```python
from build123d import *

# Parameters (mm, degrees)
F15_DEPTH = 16.5
F16_R     = 20.5
F17_DEPTH = 16.5
F18_R     = 4.0274870607
F19_DEPTH = 16.5
F20_W     = 3
F20_H     = 20
F21_DEPTH = 16.5
F22_R     = 2.75
F23_DEPTH = 40
F26_DEPTH = 31.3
F27_R     = 22.25
F28_DEPTH = 5
F29_R     = 1
F30_R     = 5
F31_R     = 5
F32_R     = 5
F33_R     = 5
F34_R     = 5
F35_R     = 2
F36_R     = 2


# Not quite as in the source:
# - a feature of the source that left no trace in its solid (it failed there, or was rolled back) is left out


with BuildPart() as f15:
    # F14 (on offset) → F15 (new body)
    with BuildSketch(Plane.XZ.offset(20)):
        Polygon((8.5, 39.5), (-8.5, 39.5365608335), (-56.3052967191, -10.4271536693), (-56.1165139079, -24.8827897012), (-50.9412027895, -33.6846895516), (12.0133129929, -33.5), (12.0133129929, -27.1025877446), (22.7434113622, -16.4029654115), (27.6456046849, 0), (22.3432332277, 17.5122059882), (8.5, 25.806048885), align=None)
    extrude(amount=F15_DEPTH)

    # F16 (on face) → F17 (cut)
    with BuildSketch(Plane.XZ.offset(36.5)):
        Circle(F16_R)
    extrude(amount=-F17_DEPTH, mode=Mode.SUBTRACT)

    # F18 (on face) → F19 (cut)
    with BuildSketch(Plane.XZ.offset(36.5)):
        with Locations((-45.0200997293, -24.5124399662)):
            Circle(F18_R)
    extrude(amount=-F19_DEPTH, mode=Mode.SUBTRACT)

    # F20 (on face) → F21 (cut)
    with BuildSketch(Plane.XZ.offset(36.5)):
        with Locations((0, 30.4450483003)):
            Rectangle(F20_W, F20_H)
    extrude(amount=-F21_DEPTH, mode=Mode.SUBTRACT)

    # F22 (on face) → F23 (cut)
    with BuildSketch(Plane.YZ.offset(8.5)):
        with Locations((-29, 32.35)):
            Circle(F22_R)
    extrude(amount=-F23_DEPTH, mode=Mode.SUBTRACT)

    # F25 (on offset) → F26 (cut)
    with BuildSketch(Plane.YZ.offset(-36.7)):
        Polygon((-32.875, 34.5872322931), (-32.875, 30.1127677069), (-29, 27.8755354138), (-25.125, 30.1127677069), (-25.125, 34.5872322931), (-29, 36.8244645862), align=None)
    extrude(amount=F26_DEPTH, mode=Mode.SUBTRACT)

    # F27 (on face) → F28 (cut)
    with BuildSketch(Plane.XZ.offset(36.5)):
        Circle(F27_R)
    extrude(amount=-F28_DEPTH, mode=Mode.SUBTRACT)

    # F29
    f29_edges = [f15.edges().sort_by_distance(p)[0] for p in [
        (-49.047587, -36.5, -24.51244),
        (-1.5, -20, 29.983277),
        (1.5, -20, 29.980051),
        (-1.5, -34, 22.199381),
        (-1.5, -31.5, 21.322214),
        (-1.5, -25.75, 20.445048),
        (1.5, -25.75, 20.445048),
        (1.5, -31.5, 21.322214),
        (1.5, -34, 22.199381),
    ]]
    fillet(f29_edges, radius=F29_R)

    # F30
    f30_edges = [f15.edges().sort_by_distance(p)[0] for p in [
        (27.645605, -28.25, 0),
    ]]
    fillet(f30_edges, radius=F30_R)

    # F31
    f31_edges = [f15.edges().sort_by_distance(p)[0] for p in [
        (22.343233, -28.25, 17.512206),
    ]]
    fillet(f31_edges, radius=F31_R)

    # F32
    f32_edges = [f15.edges().sort_by_distance(p)[0] for p in [
        (22.743411, -28.25, -16.402965),
    ]]
    fillet(f32_edges, radius=F32_R)

    # F33
    f33_edges = [f15.edges().sort_by_distance(p)[0] for p in [
        (8.5, -28.25, 25.806049),
    ]]
    fillet(f33_edges, radius=F33_R)

    # F34
    f34_edges = [f15.edges().sort_by_distance(p)[0] for p in [
        (-50.941203, -28.25, -33.68469),
        (-56.116514, -28.25, -24.88279),
        (-56.305297, -28.25, -10.427154),
    ]]
    fillet(f34_edges, radius=F34_R)

    # F35
    f35_edges = [f15.edges().sort_by_distance(p)[0] for p in [
        (12.013313, -28.25, -33.5),
        (12.013313, -28.25, -27.102588),
    ]]
    fillet(f35_edges, radius=F35_R)

    # F36
    f36_edges = [f15.edges().sort_by_distance(p)[0] for p in [
        (-8.5, -28.25, 39.536561),
        (8.5, -28.25, 39.5),
    ]]
    fillet(f36_edges, radius=F36_R)


solid = f15.part
```
Source: CAD feature listing. Evaluate the final solid. Frame: model axes, mm. A direction names the side the tool comes from. Round coordinates to 2 decimals unless told otherwise and drop trailing zeros. Write each loop counter-clockwise with the first axis right and the second up, starting at its lowest first coordinate (ties: lowest second). Pieces come first, ordered by that corner, then holes. Notation, with made-up numbers: M -3.75,62 L 43.25,62 A28 cw 43.25,95 Z; hole C 57,-14 d4. An arc over 180 degrees is marked long. Answer as a JSON object with one key per item and string values. Group by question number.
(1) Ray query, line 1 (X direction, y = -32.75, z = 34.5); line 2 (Y direction, x = 6, z = 32); line 3 (Z direction, x = -3.65, y = -29). Return the intervals inside material, ascending. Write a range as [from, to].
(2) First-contact query: pin 1 (1 mm diameter, centred on x = 10.5, y = -27.5, fed in from -Z); pin 2 (3 mm diameter, centred on y = -23, z = 0.5, fed in from +X); pin 3 (2 mm diameter, centred on y = -29.5, z = -1, fed in from -X); pin 4 (9 mm diameter, centred on y = -29, z = 32.35, fed in from +X). Flat tips, straight axial feed; report the tip coordinate or a pass-through.
(3) Reachability of faces 5 (the flat face through (-8.5, -30.91, 35.72)), 6 (the flat face through (15.877, -28.134, 21.386)), 7 (the cylindrical face through (-0.94, -34.03, -22.23)) from +Z, -Z, +X, -X, +Y, -Y: full face, straight path, thin tool, end or side. Return the list, or none.
(4) Section query A-A on x = -6.5. Output: boundary loops of the cut face in (y, z) (3 decimals).
(5) Mould query, pull axis Y, two halves, no side actions, for faces 1 (the flat face through (-8.502, -27.035, 35.69)), 2 (the cylindrical face through (27.424, -28.366, 0.02)), 3 (the flat face through (-24, -36.5, -5)), 4 (the cylindrical face through (5.049, -31.747, 32.471)). Classes: +Y half, -Y half, draft (parallel to the pull), parting line (faces both ways), or undercut.
(6) Section query B-B on z = 0. Output: boundary loops of the cut face in (x, y).
(7) Section query C-C on z = 32.35. Output: boundary loops of the cut face in (x, y) (3 decimals), then the cut area to 3 significant figures.
Computed values:
{
 "1": {"line 1": "[-5.4, -1.5], [1.5, 8.5]", "line 2": "[-36.5, -31.73], [-26.27, -20]", "line 3": "[-33.55, -20.17], [20.17, 29.6], [35.1, 39.53]"},
 "2": {"pin 1": "z = -33.51", "pin 2": "x = 27.42", "pin 3": "x = -48.24", "pin 4": "x = 8.56"},
 "3": {"face 5": "-X", "face 6": "+Z, +X, +Y, -Y", "face 7": "-Y"},
 "4": {"outline": "M -36.5,-33.554 L -20,-33.554 L -20,-19.442 L -31.5,-19.442 L -31.5,-21.279 L -36.5,-21.279 Z; M -36.5,21.279 L -31.5,21.279 L -31.5,19.442 L -20,19.442 L -20,39.532 L -36.5,39.532 Z; hole M -32.875,30.113 L -29,27.876 L -25.125,30.113 L -25.125,34.587 L -29,36.824 L -32.875,34.587 Z"},
 "5": {"face 1": "undercut", "face 2": "draft", "face 3": "-Y half", "face 4": "undercut"},
 "6": {"outline": "M -46.33,-36.5 L -22.25,-36.5 L -22.25,-31.5 L -20.5,-31.5 L -20.5,-20 L -46.33,-20 Z; M 20.5,-31.5 L 22.25,-31.5 L 22.25,-36.5 L 27.42,-36.5 L 27.42,-20 L 20.5,-20 Z"},
 "7": {"outline": "M -15.376,-36.5 L -1.5,-36.5 L -1.5,-31.75 L -5.4,-31.75 L -5.4,-32.875 L -15.376,-32.875 Z; M -15.376,-25.125 L -5.4,-25.125 L -5.4,-26.25 L -1.5,-26.25 L -1.5,-21 A1 ccw -2.5,-20 L -15.376,-20 Z; M 1.5,-36.5 L 8.5,-36.5 L 8.5,-31.75 L 1.5,-31.75 Z; M 1.5,-26.25 L 8.5,-26.25 L 8.5,-20 L 2.5,-20 A1 ccw 1.5,-21 Z", "area": "207 mm^2"}
}
